from build123d import *

# Parameters (mm, degrees)
F0_R     = 47.4803675011
F0_R_2   = 42.7485217124
F1_DEPTH = 25.4
F2_DEPTH = 18.796
F3_R     = 2.54


# Not quite as in the source:
# - a fillet or chamfer that OpenCascade refuses, or shapes differently, is made with other operations: its cross-section is extruded or revolved along the edge and cut away or added


with BuildPart() as f1:
    # F0 (on Front) → F1 (new body)
    with BuildSketch(Plane.XZ):
        Circle(F0_R)
        Circle(F0_R_2, mode=Mode.SUBTRACT)
    extrude(amount=F1_DEPTH)

    # F0 (on Front) → F2 (join)
    with BuildSketch(Plane.XZ):
        Circle(F0_R_2)
    extrude(amount=F2_DEPTH)

    # F3
    f3_edges = [f1.edges().sort_by_distance(p)[0] for p in [
        (-42.748522, -25.4, 0),
    ]]
    fillet(f3_edges, radius=F3_R)

    # F4: fillet of radius 5.08 on 1 edges, made by hand

    # F4_s1 → F4_t2 (revolve, cut)
    with BuildSketch(Plane.XY):
        with BuildLine():
            ThreePointArc((45.2885217124, -25.4), (46.8991575269, -23.5803996015), (47.4803675011, -21.2208894186))
            Line((47.4803675011, -21.2208894186), (47.4803675011, -25.4))
            Line((47.4803675011, -25.4), (45.2885217124, -25.4))
        make_face()
    revolve(axis=Axis((0, -25.4, 0), (0, -1, 0)), mode=Mode.SUBTRACT)


solid = f1.part
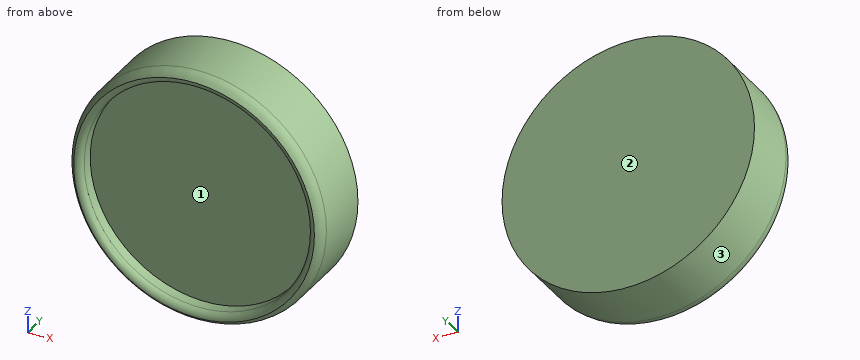
Geometry: final body of the model. Coordinates: model frame, mm. Face numbers are marked on the shaded views. Round coordinates to 2 decimals unless told otherwise and drop trailing zeros. Loops run counter-clockwise (first coordinate to the right, second up) from the corner with the lowest first, then second, coordinate; pieces in that order, holes last.
Q1. Material intervals for L1, parallel to Z at x = 0, y = -19.8; L2, parallel to Z at x = 0.5, y = -17.75; L3, parallel to Y at x = -10, z = 15.5, sorted ascending.
Q2. Section C-C on y = -4.5. Return loops of the section in (x, z).
Q3. Pin query (flat end, axial travel): P1, Ø4, axis at y = -7.5, z = 27, coming from the +X side; P2, Ø3, axis at x = -0.5, y = -18, coming from the +Z side; P3, Ø2, axis at y = -4.5, z = -31.5, coming from the -X side. Return the tip coordinate at first contact, or that it passes through.
Q4. Section A-A on z = 0. Return loops of the section in (x, y), plus the area to 3 significant figures.
Q5. Section B-B on x = 0. Return loops of the section in (y, z), plus the area to 3 significant figures.
Q6. Pull-direction query (Z, two-part tool) for the marked faces 1, 2 and 3; classes: released by +Z, released by -Z, zero draft, split by the parting line, or undercut.
Evaluation:
1. L1: z = -47.48 to -42.75, 42.75 to 47.48
1. L2: z = -47.48 to 47.48
1. L3: y = -18.8 to 0
2. outline: circle Ø94.96 at (0, 0)
3. P1: stops at x = 40.37
3. P2: stops at z = 47.48
3. P3: stops at x = -36.39
4. outline: (-47.48, -21.22) arc R5.08 ccw to (-45.29, -25.4) arc R2.54 ccw to (-42.75, -22.86) - (-42.75, -18.8) - (42.75, -18.8) - (42.75, -22.86) arc R2.54 ccw to (45.29, -25.4) arc R5.08 ccw to (47.48, -21.22) - (47.48, 0) - (-47.48, 0) - close
4. area: 1,840 mm2
5. outline: (-25.4, -45.29) arc R5.08 ccw to (-21.22, -47.48) - (0, -47.48) - (0, 47.48) - (-21.22, 47.48) arc R5.08 ccw to (-25.4, 45.29) arc R2.54 ccw to (-22.86, 42.75) - (-18.8, 42.75) - (-18.8, -42.75) - (-22.86, -42.75) arc R2.54 ccw to start
5. area: 1,840 mm2
6. face 1: undercut
6. face 2: zero draft
6. face 3: split by the parting line
